Work out the finished part from the listing and answer in its coordinate system (mm). Face numbers are marked on the shaded views. A direction names the side the tool comes from. Coordinates: 2 decimals unless noted, no trailing zeros. Order: outer loops, then holes, each group sorted by start corner. A loop starts at its lowest first (then second) coordinate and runs counter-clockwise, first axis right, second up. Notation, with made-up numbers: M -30.5,32.5 L -26.5,32.5 A14 cw -26.5,55.5 Z; hole C 61,78 d6. An arc over 180 degrees is marked long. Answer in a Markdown table with one row per item. Add a question column.
Item 1: The part is cut by section B-B (x = 33.15). Write down the section's boundary in (y, z).
Item 2: The part is cut by section A-A (z = 50). Write down the section's boundary in (x, y).
Item 3: The part is cut by section D-D (x = 44). Write down the section's boundary in (y, z).
Item 4: Consider line 1 (X direction, y = 6.5, z = 18.5); line 2 (X direction, y = 1.6, z = 50); line 3 (Z direction, x = 37, y = 7.5). Determine where each line is inside the solid, lowest interval first. Write a range as from..to.
Item 5: Flat-ended cylindrical pins translate along their axes: pin 1 Ø4 at (x, y) = (43.5, 8) entering from -Z; pin 2 Ø2 at (x, z) = (8, 39.5) entering from +Y; pin 3 Ø15 at (x, z) = (34.5, 33) entering from +Y; pin 4 Ø3.5 at (x, z) = (33.15, 50) entering from -Y. Find the tip coordinate at first contact, or state that the pin passes through.
Item 6: The mould has two halves that part along X. Classify the marked faces 4, 5 and 6: released by +X, released by -X, zero draft, split by the parting line, or undercut.
Item 7: Which of the six approach directions +Z, -Z, +X, -X, +Y, -Y give full straight-line access (tool end or side, diameter ignored) to the marked faces 1, 2 and 3?
Item 8: The part is cut by section C-C (z = 42.5). Write down the section's boundary in (x, y), then the cut area to 3 significant figures.
from build123d import *

# Parameters (mm, degrees)
SKETCH_1_W      = 66.3
SKETCH_1_H      = 3
BASE_DEPTH      = 60
RAILS_DEPTH     = 60
SKETCH_3_R      = 2
HOLES_DEPTH     = 90.775776243
CHAMFER_1_SIZE  = 2
CHAMFER_1_SIZE2 = 1
SKETCH_4_W      = 66.3
SKETCH_4_H      = 11
FLOOR_2_DEPTH   = 3
SKETCH_5_W      = 10
SKETCH_5_H      = 5
EXTRUDE_1_DEPTH = 5
FILLET_1_R      = 10


with BuildPart() as part:
    # Эскиз1 → base (new body)
    with BuildSketch(Plane.XY):
        with Locations((33.15, 1.5)):
            Rectangle(SKETCH_1_W, SKETCH_1_H)
    extrude(amount=BASE_DEPTH)

    # Эскиз2 → rails (add)
    with BuildSketch(Plane.XY):
        Polygon((0, 3), (10, 3), (10, 6), (3, 6), (3, 8), (10, 8), (10, 11), (0, 11), align=None)
        Polygon((56.3, 11), (56.3, 8), (63.3, 8), (63.3, 6), (56.3, 6), (56.3, 3), (66.3, 3), (66.3, 11), align=None)
    extrude(amount=RAILS_DEPTH)

    # Эскиз3 → holes (cut, through all)
    with BuildSketch(Plane(origin=(0, 3, 0), x_dir=(1, 0, 0), z_dir=(0, 1, 0))):
        with Locations(Location((33.15, -10, 0), (0, 0, 270))):
            Circle(SKETCH_3_R)
        with Locations(Location((33.15, -50, 0), (0, 0, 270))):
            Circle(SKETCH_3_R)
    extrude(amount=-HOLES_DEPTH, mode=Mode.SUBTRACT)

    # Фаска1
    chamfer_1_edges = [part.edges().sort_by_distance(p)[0] for p in [
        (33.15, 3, 8),
        (33.15, 3, 48),
    ]]
    chamfer_1_side = [part.faces().sort_by_distance(p)[0] for p in [
        (33.15, 3, 30),
    ]]
    chamfer(chamfer_1_edges, length=CHAMFER_1_SIZE, length2=CHAMFER_1_SIZE2, reference=chamfer_1_side[0])

    # Эскиз4 → floor 2 (add)
    with BuildSketch(Plane.XY.offset(60)):
        with Locations((33.15, 5.5)):
            Rectangle(SKETCH_4_W, SKETCH_4_H)
    extrude(amount=FLOOR_2_DEPTH)

    # Эскиз5 → Вытянуть1 (add)
    with BuildSketch(Plane(origin=(0, 11, 0), x_dir=(1, 0, 0), z_dir=(0, 1, 0))):
        with Locations((5, -2.5)):
            Rectangle(SKETCH_5_W, SKETCH_5_H)
        with Locations((61.3, -2.5)):
            Rectangle(SKETCH_5_W, SKETCH_5_H)
    extrude(amount=EXTRUDE_1_DEPTH)

    # Скругление1
    # the kernel refuses this fillet: 10 mm, written as the material it adds along each edge
    with BuildSketch(Plane(origin=(56.3, 11, 5), x_dir=(0, 0, 1), z_dir=(1, 0, 0))) as fillet_1_piece_1:
        with BuildLine():
            CenterArc((8.660254038, -10), FILLET_1_R, 90, 60)
            Line((0, -5), (-0.173205081, -4.9))
            ThreePointArc((-0.173205081, -4.9), (-0.2, -2.5), (-0.2, 0))
            Line((-0.2, 0), (0, 0.2))
            Line((0, 0.2), (8.660254038, 0.2))
            Line((8.660254038, 0.2), (8.660254038, 0))
        make_face()
    extrude(amount=10)
    with BuildSketch(Plane(origin=(10, 11, 5), x_dir=(0, 0, 1), z_dir=(-1, 0, 0))) as fillet_1_piece_2:
        with BuildLine():
            CenterArc((8.660254038, 10), FILLET_1_R, 210, 60)
            Line((0, 5), (-0.173205081, 4.9))
            ThreePointArc((-0.173205081, 4.9), (-0.2, 2.5), (-0.2, 0))
            Line((-0.2, 0), (0, -0.2))
            Line((0, -0.2), (8.660254038, -0.2))
            Line((8.660254038, -0.2), (8.660254038, 0))
        make_face()
    extrude(amount=10)


solid = part.part
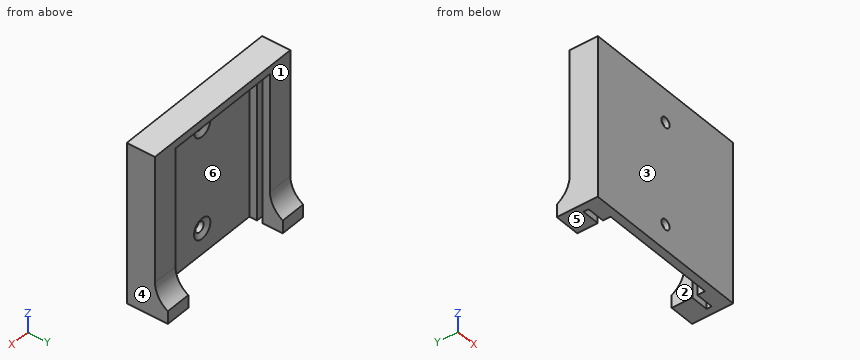
Reply:
| question | item | result |
|---|---|---|
| 1 | outline | M 0,0 L 3,0 L 3,6 L 2,8 L 0,8 Z; M 0,12 L 2,12 L 3,14 L 3,46 L 2,48 L 0,48 Z; M 0,52 L 2,52 L 3,54 L 3,60 L 11,60 L 11,63 L 0,63 Z |
| 2 | outline | M 0,0 L 31.15,0 L 31.15,2 L 29.15,3 L 10,3 L 10,6 L 3,6 L 3,8 L 10,8 L 10,11 L 0,11 Z; M 35.15,0 L 66.3,0 L 66.3,11 L 56.3,11 L 56.3,8 L 63.3,8 L 63.3,6 L 56.3,6 L 56.3,3 L 37.15,3 L 35.15,2 Z |
| 3 | outline | M 0,0 L 3,0 L 3,60 L 11,60 L 11,63 L 0,63 Z |
| 4 | line 1 | x = 0..3, 63.3..66.3 |
| 4 | line 2 | x = 0..31.15, 35.15..66.3 |
| 4 | line 3 | z = 60..63 |
| 5 | pin 1 | stops at z = 60 |
| 5 | pin 2 | stops at y = 11 |
| 5 | pin 3 | stops at y = 3 |
| 5 | pin 4 | passes through |
| 6 | face 4 | released by +X |
| 6 | face 5 | zero draft |
| 6 | face 6 | undercut |
| 7 | face 1 | +Z, +X, -X, +Y |
| 7 | face 2 | -Z, +Y |
| 7 | face 3 | +Z, -Z, +X, -X, -Y |
| 8 | outline | M 0,0 L 66.3,0 L 66.3,11 L 56.3,11 L 56.3,8 L 63.3,8 L 63.3,6 L 56.3,6 L 56.3,3 L 10,3 L 10,6 L 3,6 L 3,8 L 10,8 L 10,11 L 0,11 Z |
| 8 | area | 331 mm2 |
